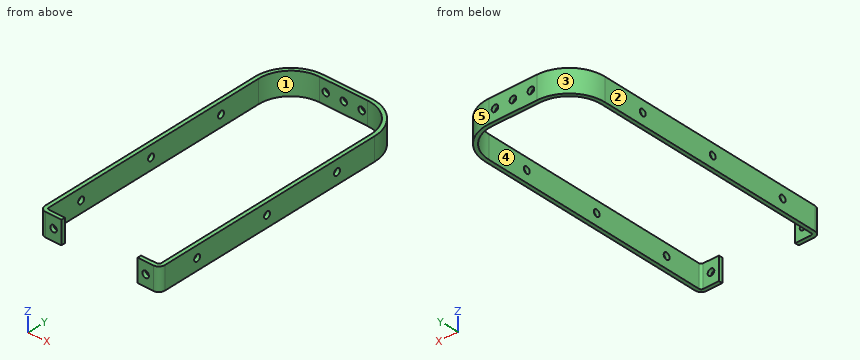
from build123d import *

# Parameters (mm, degrees)
BOSS_EXTRUDE1_DEPTH     = 9.525
SKETCH12_R              = 2.75
CUT_EXTRUDE2_DEPTH      = 236.564695201
CUT_EXTRUDE3_DEPTH      = 289.081109455
CUT_EXTRUDE3_DEPTH_BACK = 289.081109455
SKETCH13_R              = 2.75
CUT_EXTRUDE6_REACH      = 237.565
SKETCH16_R              = 2.75


with BuildPart() as part:
    # Sketch1 → Boss-Extrude1 (new, symmetric)
    with BuildSketch(Plane.XY):
        with BuildLine():
            Line((50, 45), (50, 240))
            ThreePointArc((50, 240), (41.213203436, 261.213203436), (20, 270))
            Line((20, 270), (-20, 270))
            ThreePointArc((-20, 270), (-41.213203436, 261.213203436), (-50, 240))
            Line((-50, 240), (-50, 45))
            ThreePointArc((-50, 45), (-48.535533906, 41.464466094), (-45, 40))
            Line((-45, 40), (-31.825, 40))
            Line((-31.825, 40), (-31.825, 43.175))
            Line((-31.825, 43.175), (-45, 43.175))
            ThreePointArc((-45, 43.175), (-46.290469876, 43.709530124), (-46.825, 45))
            Line((-46.825, 45), (-46.825, 240))
            ThreePointArc((-46.825, 240), (-38.968139405, 258.968139405), (-20, 266.825))
            Line((-20, 266.825), (20, 266.825))
            ThreePointArc((20, 266.825), (38.968139405, 258.968139405), (46.825, 240))
            Line((46.825, 240), (46.825, 45))
            ThreePointArc((46.825, 45), (46.290469876, 43.709530124), (45, 43.175))
            Line((45, 43.175), (31.825, 43.175))
            Line((31.825, 43.175), (31.825, 40))
            Line((31.825, 40), (45, 40))
            ThreePointArc((45, 40), (48.535533906, 41.464466094), (50, 45))
        make_face()
    extrude(amount=BOSS_EXTRUDE1_DEPTH, both=True)

    # Sketch12 → Cut-Extrude2 (cut, through all)
    with BuildSketch(Plane(origin=(0, 270, 0), x_dir=(1, 0, 0), z_dir=(0, 1, 0))):
        with Locations(Location((0, 0, 0), (0, 0, 270))):
            Circle(SKETCH12_R)
        with Locations(Location((-15, 0, 0), (0, 0, 270))):
            Circle(SKETCH12_R)
        with Locations(Location((15, 0, 0), (0, 0, 270))):
            Circle(SKETCH12_R)
    extrude(amount=-CUT_EXTRUDE2_DEPTH, mode=Mode.SUBTRACT)

    # Sketch13 → Cut-Extrude3 (cut, two sides: drawn at the far end of the back side and taken through both)
    with BuildSketch(Plane(origin=(50, 0, 0), x_dir=(0, 0, -1), z_dir=(1, 0, 0)).offset(-CUT_EXTRUDE3_DEPTH_BACK)):
        with Locations(Location((0, 205, 0), (0, 0, 90))):
            Circle(SKETCH13_R)
        with Locations(Location((0, 140, 0), (0, 0, 90))):
            Circle(SKETCH13_R)
        with Locations(Location((0, 75, 0), (0, 0, 90))):
            Circle(SKETCH13_R)
    extrude(amount=CUT_EXTRUDE3_DEPTH + CUT_EXTRUDE3_DEPTH_BACK, mode=Mode.SUBTRACT)

    # Sketch16 → Cut-Extrude6 (cut, up to next)
    with BuildSketch(Plane(origin=(0, 40, 0), x_dir=(-1, 0, 0), z_dir=(0, -1, 0)), mode=Mode.PRIVATE) as cut_extrude6_sk1:
        with Locations(Location((38.4125, 0, 0), (0, 0, 180))):
            Circle(SKETCH16_R)
    cut_extrude6_tool1 = extrude(cut_extrude6_sk1.sketch, amount=-CUT_EXTRUDE6_REACH, mode=Mode.PRIVATE) & part.part
    # Sketch16 → Cut-Extrude6 (cut, up to next)
    with BuildSketch(Plane(origin=(0, 40, 0), x_dir=(-1, 0, 0), z_dir=(0, -1, 0)), mode=Mode.PRIVATE) as cut_extrude6_sk2:
        with Locations(Location((-38.4125, 0, 0), (0, 0, 180))):
            Circle(SKETCH16_R)
    cut_extrude6_tool2 = extrude(cut_extrude6_sk2.sketch, amount=-CUT_EXTRUDE6_REACH, mode=Mode.PRIVATE) & part.part
    add(cut_extrude6_tool1.solids().sort_by_distance((-38.4125, 40, 0))[0], mode=Mode.SUBTRACT)
    add(cut_extrude6_tool2.solids().sort_by_distance((38.4125, 40, 0))[0], mode=Mode.SUBTRACT)


solid = part.part
Here's how the part is built. I have some questions about the finished solid (model axes, mm). Face numbers are marked on the shaded views. A direction names the side the tool comes from. Give positions to 0.01 mm unless a question says otherwise; leave off trailing zeros. Loops run counter-clockwise (first coordinate to the right, second up) from the corner with the lowest first, then second, coordinate; pieces in that order, holes last. Notation, with made-up numbers: (0, -26) -> (28, -26) arc R31 ccw to (28, 13) -> close; hole circle Ø7 at (22, -34). An arc over 180 degrees is marked (long way). Answer as a JSON object with one key per item and string values. Group by question number.
Item 1: I need wall thicknesses on L1, parallel to Z at x = -48.4, y = 205 (3 decimals); L2, parallel to X at y = 221, z = -4.5 (3 decimals); L3, parallel to Y at x = -32, z = 3.75 (3 decimals). Which ranges of each line are inside material? Lowest first, please.
Item 2: Imagine slicing it at C-C on y = 135. Write out the boundary of the cut face in (x, z) (3 decimals).
Item 3: Will these pins go through, and if not, where does the flat tip stop? pin 1 (3.5 mm diameter, centred on y = 41, z = 3.5, fed in from +X); pin 2 (6 mm diameter, centred on x = 35, z = 0.5, fed in from +Y); pin 3 (6.5 mm diameter, centred on y = 205, z = 0, fed in from +X); pin 4 (4 mm diameter, centred on x = -36, z = 4, fed in from +Y).
Item 4: On a 3-axis mill with a long thin cutter (end or side, diameter ignored), from which of +Z, -Z, +X, -X, +Y, -Y can I reach the whole of each face in a straight line? I mean the marked faces 1 and 2. Say none if no direction works.
Item 5: Imagine slicing it at B-B on y = 75. Write out the boundary of the cut face in (x, z) (3 decimals), then the cut area to 3 significant figures.
Item 6: Thinking about a two-plate mould opening in X: for the marked faces 3, 4 and 5, which applies, pulls with the +X half, pulls with the -X half, needs draft (parallel to the pull), parting line crosses it, or undercut?
Item 7: Imagine slicing it at A-A on x = 15. Write out the boundary of the cut face in (y, z) (3 decimals), then the cut area to 3 significant figures.
Answer list:
{
 "1": {"L1": "z = -9.525 to -2.75, 2.75 to 9.525", "L2": "x = -50 to -46.825, 46.825 to 50", "L3": "y = 40 to 43.175, 263.991 to 267.495"},
 "2": {"outline": "(-50, -9.525) -> (-46.825, -9.525) -> (-46.825, 9.525) -> (-50, 9.525) -> close; (46.825, -9.525) -> (50, -9.525) -> (50, 9.525) -> (46.825, 9.525) -> close"},
 "3": {"pin 1": "stops at x = 49.47", "pin 2": "stops at y = 267.5", "pin 3": "stops at x = 50", "pin 4": "stops at y = 266.53"},
 "4": {"face 1": "+Z, -Z", "face 2": "+Z, -Z, -X, +Y, -Y"},
 "5": {"outline": "(-50, -9.525) -> (-46.825, -9.525) -> (-46.825, -2.75) -> (-50, -2.75) -> close; (-50, 2.75) -> (-46.825, 2.75) -> (-46.825, 9.525) -> (-50, 9.525) -> close; (46.825, -9.525) -> (50, -9.525) -> (50, -2.75) -> (46.825, -2.75) -> close; (46.825, 2.75) -> (50, 2.75) -> (50, 9.525) -> (46.825, 9.525) -> close", "area": "86.0 mm2"},
 "6": {"face 3": "pulls with the -X half", "face 4": "undercut", "face 5": "pulls with the +X half"},
 "7": {"outline": "(266.825, -9.525) -> (270, -9.525) -> (270, -2.75) -> (266.825, -2.75) -> close; (266.825, 2.75) -> (270, 2.75) -> (270, 9.525) -> (266.825, 9.525) -> close", "area": "43.0 mm2"}
}
